Geometry check sheet. Reference: the model listing, model coordinates, mm. Face numbers are marked on the shaded views. A direction names the side the tool comes from. Round coordinates to 2 decimals unless told otherwise and drop trailing zeros. Order: outer loops, then holes, each group sorted by start corner. A loop starts at its lowest first (then second) coordinate and runs counter-clockwise, first axis right, second up. Notation, with made-up numbers: (-21.5, 1.25) - (14.5, 1.25) arc R25 cw to (14.5, 36.25) - close; hole circle Ø2 at (22.25, 81.5). An arc over 180 degrees is marked (long way). Use a Markdown table: item, result. Add a question column.
(1) Thickness scan on line 1 along X through (y, z) = (20.5, 11.75); line 2 along Y through (x, z) = (11, 14). Record the ranges inside material, lowest first. Write a range as [from, to].
(2) Section check A-A on y = 18. Record the boundary of the cut face in (x, z), then the cut area to 3 significant figures.
(3) Mould release check, pull along X, two halves, no side actions. Record for the marked faces 1, 2 and 3: released by +X, released by -X, zero draft, split by the parting line, or undercut.
(4) Gauge pin test, flat ends, axial feed: P1, Ø4, axis at y = 13, z = 7.5, coming from the -X side; P2, Ø4.5, axis at x = 19, z = 9.5, coming from the -Y side. Record the tip position at first contact, or that the pin passes through.
(5) Section check C-C on x = 12.5. Record the boundary of the cut face in (y, z).
(6) Access from +Z, -Z, +X, -X, +Y, -Y to the whole of each face (thin tool, end or side, straight path). Record for the marked faces 4 and 5.
(7) Section check B-B on z = 3.25. Record the boundary of the cut face in (x, y), then the cut area to 3 significant figures.
```python
from build123d import *

# Parameters (mm, degrees)
F0_W     = 50
F0_H     = 15
F1_DEPTH = 40
F2_W     = 20
F2_H     = 25
F3_DEPTH = 25


with BuildPart() as f1:
    # F0 (on Right) → F1 (new body)
    with BuildSketch(Plane.YZ):
        with Locations((25, 7.5)):
            Rectangle(F0_W, F0_H)
    extrude(amount=F1_DEPTH)

    # F2 (on face) → F3 (cut)
    with BuildSketch(Plane.XY.offset(15)):
        with Locations((20, 12.5)):
            Rectangle(F2_W, F2_H)
    extrude(amount=-F3_DEPTH, mode=Mode.SUBTRACT)


solid = f1.part
```
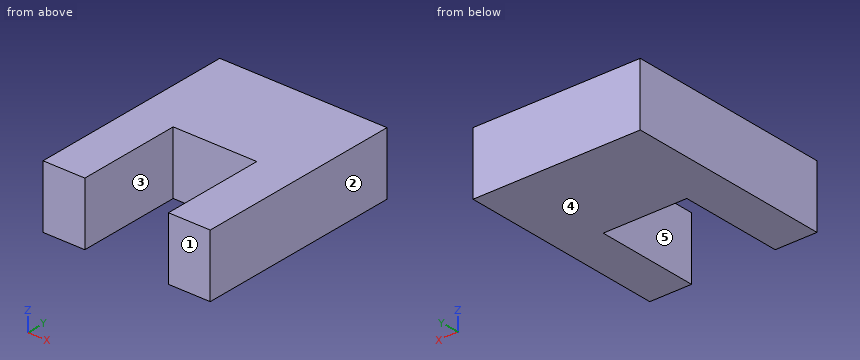
Check sheet entries:
| question | item | result |
|---|---|---|
| 1 | line 1 | x = [0, 10], [30, 40] |
| 1 | line 2 | y = [25, 50] |
| 2 | outline | (0, 0) - (10, 0) - (10, 15) - (0, 15) - close; (30, 0) - (40, 0) - (40, 15) - (30, 15) - close |
| 2 | area | 300 mm2 |
| 3 | face 1 | zero draft |
| 3 | face 2 | released by +X |
| 3 | face 3 | undercut |
| 4 | P1 | stops at x = 0 |
| 4 | P2 | stops at y = 25 |
| 5 | outline | (25, 0) - (50, 0) - (50, 15) - (25, 15) - close |
| 6 | face 4 | -Z, +X, -X, +Y, -Y |
| 6 | face 5 | +Z, -Z, -Y |
| 7 | outline | (0, 0) - (10, 0) - (10, 25) - (30, 25) - (30, 0) - (40, 0) - (40, 50) - (0, 50) - close |
| 7 | area | 1,500 mm2 |
